Can you work these out from the model? Positions are in its coordinate system, mm. A direction names the side the tool comes from. Round coordinates to 2 decimals unless told otherwise and drop trailing zeros. Loops run counter-clockwise (first coordinate to the right, second up) from the corner with the lowest first, then second, coordinate; pieces in that order, holes last. Notation, with made-up numbers: (-9, 45) -> (7, 45) arc R21 ccw to (7, 54) -> close; hole circle Ø4 at (29.25, -11). An arc over 180 degrees is marked (long way). Write item = value, one per line.
from build123d import *

# Parameters (mm, degrees)
EXTRUDE_1_DEPTH     = 3
SKETCH_2_R          = 1.575
CUT_EXTRUDE_1_DEPTH = 54.235326617
FILLET_1_R          = 2
FILLET_2_R          = 5


with BuildPart() as part:
    # 草图1 → 凸台-拉伸1 (new body)
    with BuildSketch(Plane.XY):
        Polygon((0, 0), (20, 0), (40, -20), (40, -35), (-20, -35), (-20, -20), align=None)
    extrude(amount=EXTRUDE_1_DEPTH)

    # 草图2 → 切除-拉伸1 (cut, through all)
    with BuildSketch(Plane.XY.offset(3)):
        with Locations((5, -5)):
            Circle(SKETCH_2_R)
        with Locations(Location((15, -5, 0), (0, 0, 180))):
            Circle(SKETCH_2_R)
        with Locations((15, -15)):
            Circle(SKETCH_2_R)
        with Locations(Location((5, -15, 0), (0, 0, 180))):
            Circle(SKETCH_2_R)
        with Locations((-15, -31.5)):
            Circle(SKETCH_2_R)
        with Locations(Location((-15, -23.5, 0), (0, 0, 180))):
            Circle(SKETCH_2_R)
        with Locations(Location((-5, -31.5, 0), (0, 0, 180))):
            Circle(SKETCH_2_R)
        with Locations((-5, -23.5)):
            Circle(SKETCH_2_R)
        with Locations((25, -31.5)):
            Circle(SKETCH_2_R)
        with Locations(Location((35, -31.5, 0), (0, 0, 180))):
            Circle(SKETCH_2_R)
        with Locations(Location((25, -23.5, 0), (0, 0, 180))):
            Circle(SKETCH_2_R)
        with Locations((35, -23.5)):
            Circle(SKETCH_2_R)
        Polygon((0, -5.656854249), (0, -20), (-14.343145751, -20), align=None)
        Polygon((34.343145751, -20), (20, -5.656854249), (20, -20), align=None)
    extrude(amount=-CUT_EXTRUDE_1_DEPTH, mode=Mode.SUBTRACT)

    # 圆角1
    fillet_1_edges = [part.edges().sort_by_distance(p)[0] for p in [
        (34.343145751, -20, 1.5),
        (20, -20, 1.5),
        (20, -5.656854249, 1.5),
        (-14.343145751, -20, 1.5),
        (0, -5.656854249, 1.5),
        (0, -20, 1.5),
    ]]
    fillet(fillet_1_edges, radius=FILLET_1_R)

    # 圆角2
    fillet_2_edges = [part.edges().sort_by_distance(p)[0] for p in [
        (0, 0, 1.5),
        (20, 0, 1.5),
        (40, -20, 1.5),
        (40, -35, 1.5),
        (-20, -35, 1.5),
        (-20, -20, 1.5),
    ]]
    fillet(fillet_2_edges, radius=FILLET_2_R)


solid = part.part
1. Suppose I cut it at D-D, the plane x = -5. List the corners of the cut face in (y, z) for me (3 decimals).
Entries:
outline = (-35, 0) -> (-33.075, 0) -> (-33.075, 3) -> (-35, 3) -> close; (-29.925, 0) -> (-25.075, 0) -> (-25.075, 3) -> (-29.925, 3) -> close; (-21.925, 0) -> (-20, 0) -> (-20, 3) -> (-21.925, 3) -> close; (-10.657, 0) -> (-5, 0) -> (-5, 3) -> (-10.657, 3) -> close
2. Suppose I cut it at A-A, the plane x = 15. List the corners of the cut face in (y, z) for me (3 decimals), and give its area (3 significant figures).
Entries:
outline = (-35, 0) -> (-16.575, 0) -> (-16.575, 3) -> (-35, 3) -> close; (-13.425, 0) -> (-6.575, 0) -> (-6.575, 3) -> (-13.425, 3) -> close; (-3.425, 0) -> (0, 0) -> (0, 3) -> (-3.425, 3) -> close
area = 86.1 mm²
3. I need wall thicknesses on line 1 (Y direction, x = -15, z = 2.15) (3 decimals); line 2 (Y direction, x = 15, z = 1.7) (3 decimals); line 3 (X direction, y = -23, z = 1.4). Which ranges of each line are inside material? Lowest first, please. Write a range as [from, to].
Entries:
line_1 = [-35, -33.075], [-29.925, -25.075], [-21.925, -15]
line_2 = [-35, -16.575], [-13.425, -6.575], [-3.425, 0]
line_3 = [-20, -16.49], [-13.51, -6.49], [-3.51, 23.51], [26.49, 33.51], [36.49, 40]
4. For faces 5 (the cylindrical face through (-0.6, -19.43, 1.48)), 6 (the cylindrical face through (39, -33, 2)), which set-ups out of +Z, -Z, +X, -X, +Y, -Y let a thin tool reach every point of the face, with its end or its side?
Entries:
face_5 = +Z, -Z
face_6 = +Z, -Z, +X, -Y
5. Suppose I cut it at C-C, the plane z = 1.9. Count the separate pieces of the cut face and the enclosed holes in it, and give its area (3 significant figures).
Entries:
separate_pieces = 1
enclosed_holes = 14
area = 1,410 mm²
6. We'd pull the mould along X, two halves only. Please class faces 1 (the flat face through (26, -20, 2)), 2 (the cylindrical face through (39.61, -20.13, 1.52)), 3 (the flat face through (-10, -10, 1)), 4 (the cylindrical face through (-5.341, -25.038, 1.521)): released by +X, released by -X, zero draft, split by the parting line, or undercut.
Entries:
face_1 = undercut
face_2 = released by +X
face_3 = released by -X
face_4 = undercut
7. I'm going to push flat-ended pins straight in: pin 1 (0.9 mm diameter, centred on x = -7, z = 2, fed in from +Y); pin 2 (1.5 mm diameter, centred on y = -15.5, z = 1, fed in from -X). Where does each tip first touch, or does it pass through?
Entries:
pin_1 = -6.55
pin_2 = -16.25
8. Suppose I cut it at B-B, the plane y = -31.5. List the corners of the cut face in (x, z) for me (3 decimals), and give its area (3 significant figures).
Entries:
outline = (-19.77, 0) -> (-16.575, 0) -> (-16.575, 3) -> (-19.77, 3) -> close; (-13.425, 0) -> (-6.575, 0) -> (-6.575, 3) -> (-13.425, 3) -> close; (-3.425, 0) -> (23.425, 0) -> (23.425, 3) -> (-3.425, 3) -> close; (26.575, 0) -> (33.425, 0) -> (33.425, 3) -> (26.575, 3) -> close; (36.575, 0) -> (39.77, 0) -> (39.77, 3) -> (36.575, 3) -> close
area = 141 mm²
